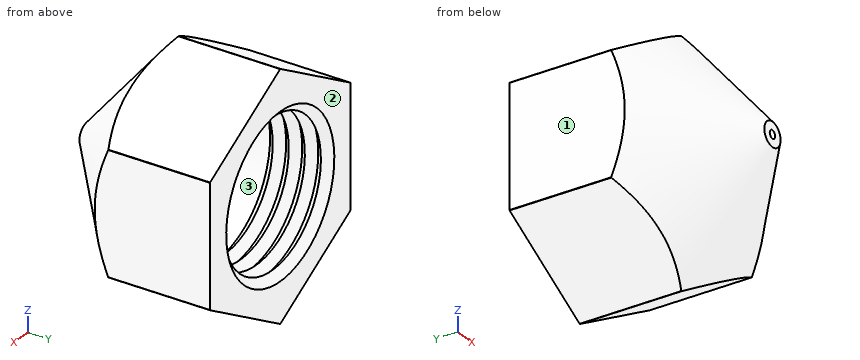
from build123d import *

# Parameters (mm, degrees)
SKETCH2_OUTSIDE_W  = 21.874
SKETCH2_OUTSIDE_H  = 21.874
CUT_EXTRUDE1_DEPTH = 13


with BuildPart() as part:
    # Sketch1 → Revolve1 (revolve)
    with BuildSketch(Plane.XY, mode=Mode.PRIVATE) as revolve1_sk:
        Polygon((0.25, -12), (0.75, -12), (7.5, -6.33607749), (7.5, 0), (5, 0), (4.5, -0.5), (5, -1), (4.5, -1.5), (5, -2), (4.5, -2.5), (5, -3), (4.5, -3.5), (5, -4), (5, -6), (2.0875, -6), (1.5875, -6.5), (1.5875, -9.90602957), (0.25, -11.5), align=None)
    revolve(revolve1_sk.sketch.rotate(Axis((0, 0, 0), (0, -1, 0)), 90), axis=Axis((0, 0, 0), (0, -1, 0)))  # turned: the seam where the file's is

    # Sketch2 outside → Cut-Extrude1 (cut, through all)
    with BuildSketch(Plane(origin=(0, 0, 0), x_dir=(1, 0, 0), z_dir=(0, 1, 0))):
        Rectangle(SKETCH2_OUTSIDE_W, SKETCH2_OUTSIDE_H)
        Polygon((0, 7.505553499), (-6.5, 3.75277675), (-6.5, -3.75277675), (0, -7.505553499), (6.5, -3.75277675), (6.5, 3.75277675), align=None, mode=Mode.SUBTRACT)
    extrude(amount=-CUT_EXTRUDE1_DEPTH, mode=Mode.SUBTRACT)


solid = part.part
Design review of the part built by this model. Coordinates are the model's own, in mm. Face numbers are marked on the shaded views. Round coordinates to 2 decimals unless told otherwise and drop trailing zeros. Loops run counter-clockwise (first coordinate to the right, second up) from the corner with the lowest first, then second, coordinate; pieces in that order, holes last. Notation, with made-up numbers: (-17, 41.25) - (10, 41.25) arc R29 cw to (10, 71.25) - close; hole circle Ø8 at (43.5, 49.5). An arc over 180 degrees is marked (long way). One line per item, written item: value. Start each with the question number.
1) To check wall thickness, follow L1, parallel to X at y = -8.6, z = 0; L2, parallel to Z at x = 4.25, y = -5.5; L3, parallel to X at y = -7.3, z = 0. State the ranges of each line that lie inside material, in increasing order. Write a range as from..to.
2) Consider section C-C on y = -7.5. Give the boundary of the cut face in (x, z) (1 decimal), then the cut area to 3 significant figures.
3) Insertion check: pin 1 Ø2 at (x, z) = (-1.5, 5) entering from -Y; pin 2 Ø4 at (x, z) = (0, 0) entering from +Y; pin 3 Ø3 at (x, z) = (2.5, 0) entering from +Y; pin 4 Ø3 at (x, z) = (2, 3) entering from +Y. Each pin has a flat end and moves straight along its axis. Give the tip position at first contact, or say it passes through.
4) Consider section B-B on y = -10.75. Give the boundary of the cut face in (x, z), then the cut area to 3 significant figures.
5) Draft analysis for pull direction X (two halves, no side actions). For the marked faces 1, 2 and 3, state which applies: +X half, -X half, draft (parallel to the pull), parting line (faces both ways), or undercut.
Reported:
1. L1: x = -4.8..-1.59, 1.59..4.8
1. L2: z = -5.05..-2.63, 2.63..5.05
1. L3: x = -6.35..-1.59, 1.59..6.35
2. outline: circle Ø12.2 at (0, 0); hole circle Ø3.2 at (0, 0)
2. area: 109 mm^2
3. pin 1: stops at y = -9.09
3. pin 2: stops at y = -6.09
3. pin 3: stops at y = -6
3. pin 4: stops at y = 0
4. outline: circle Ø4.48 at (0, 0); hole circle Ø1.76 at (0, 0)
4. area: 13.3 mm^2
5. face 1: -X half
5. face 2: draft
5. face 3: undercut
